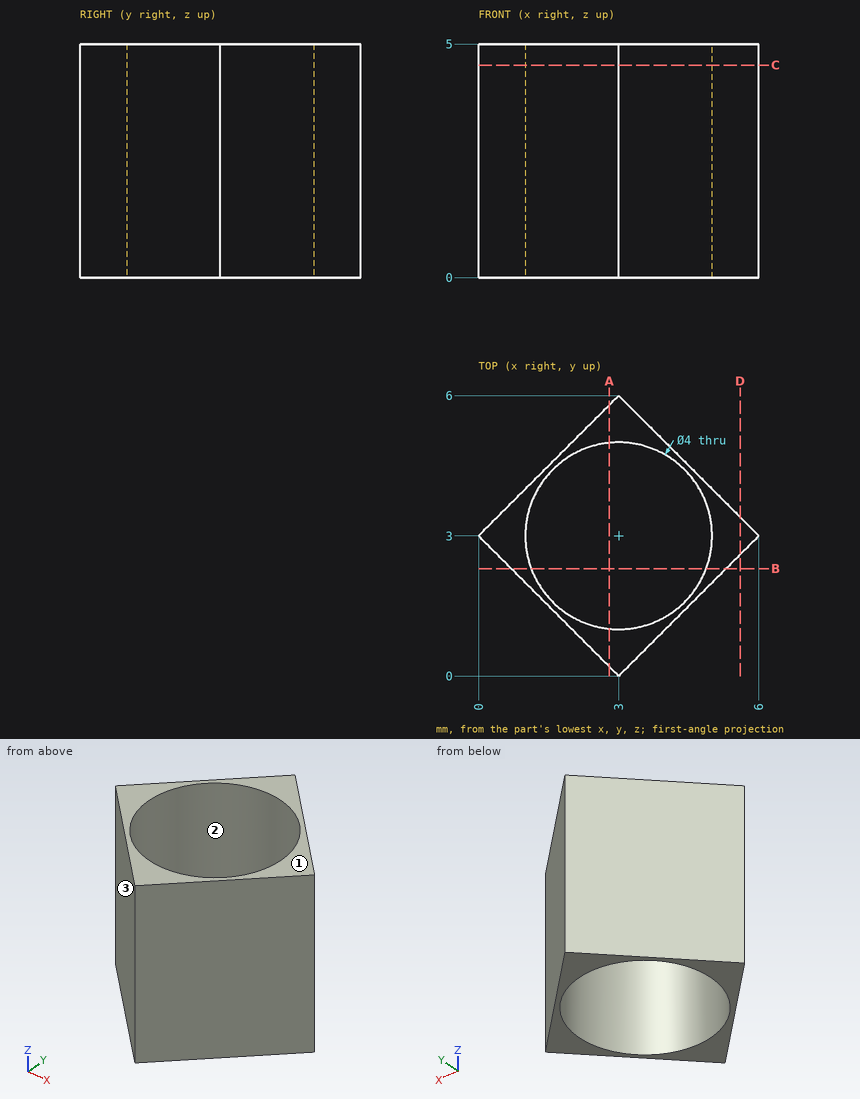
Check sheet for the drawn part. Datum: minimum x, y, z corner. Units: mm. Round coordinates to 2 decimals unless told otherwise and drop trailing zeros. Order: outer loops, then holes, each group sorted by start corner. A loop starts at its lowest first (then second) coordinate and runs counter-clockwise, first axis right, second up. Notation, with made-up numbers: (-5.75, -37) -> (20.25, -37) arc R16 cw to (20.25, -7) -> close; hole circle Ø6 at (40, 40). An arc over 180 degrees is marked (long way). Put each result on its own line as item: value. Start each with the question number.
(1) Section check B-B (y = 2.3). Enter the section's corners in (x, z), then the cut area to 4 significant figures.
(2) Material ranges on line 1 along Y through (x, z) = (4.15, 3.3); line 2 along X through (y, z) = (2.6, 2.1); line 3 along X through (y, z) = (1.55, 2), recorded low to high.
(3) Section check A-A (x = 2.8). Enter the section's corners in (y, z), then the cut area to 3 significant figures.
(4) Depth check by flat-ended pin: pin 1 Ø2 at (x, y) = (2.5, 4) entering from -Z; pin 2 Ø2 at (x, z) = (1.5, 4) entering from +Y; pin 3 Ø3 at (y, z) = (2, 1.5) entering from +X; pin 4 Ø2.5 at (x, y) = (3, 3) entering from -Z. Enter the tip coordinate at first touch or a pass-through.
(5) Section check D-D (x = 5.6). Enter the section's corners in (y, z), then the cut area to 3 significant figures.
(6) Section check C-C (z = 4.55). Enter the section's corners in (x, y), then the cut area to 3 significant figures.
(7) Draft check along Y on the marked faces 1, 2 and 3. Enter one of: +Y half, -Y half, draft (parallel to the pull), parting line (faces both ways), or undercut.
Completed:
1. outline: (0.7, 0) -> (1.13, 0) -> (1.13, 5) -> (0.7, 5) -> close; (4.87, 0) -> (5.3, 0) -> (5.3, 5) -> (4.87, 5) -> close
1. area: 4.265 mm2
2. line 1: y = 1.15 to 1.36, 4.64 to 4.85
2. line 2: x = 0.4 to 1.04, 4.96 to 5.6
2. line 3: x = 1.45 to 1.62, 4.38 to 4.55
3. outline: (0.2, 0) -> (1.01, 0) -> (1.01, 5) -> (0.2, 5) -> close; (4.99, 0) -> (5.8, 0) -> (5.8, 5) -> (4.99, 5) -> close
3. area: 8.10 mm2
4. pin 1: stops at z = 0
4. pin 2: stops at y = 5.5
4. pin 3: stops at x = 6
4. pin 4: passes through
5. outline: (2.6, 0) -> (3.4, 0) -> (3.4, 5) -> (2.6, 5) -> close
5. area: 4.00 mm2
6. outline: (0, 3) -> (3, 0) -> (6, 3) -> (3, 6) -> close; hole circle Ø4 at (3, 3)
6. area: 5.43 mm2
7. face 1: draft
7. face 2: undercut
7. face 3: -Y half
